Geometry: final body of the model. Coordinates: model frame, mm. A direction names the side the tool comes from. Give positions to 0.01 mm unless a question says otherwise; leave off trailing zeros. Loops run counter-clockwise (first coordinate to the right, second up) from the corner with the lowest first, then second, coordinate; pieces in that order, holes last. Notation, with made-up numbers: M 75.5,9 L 132.5,9 A4 ccw 132.5,15 Z; hole C -13.75,43 d10. An arc over 180 degrees is marked long. Put each result on its own line as item: value.
Autodesk Fusion 360 part; units mm, degrees
sketch "Sketch1" plane through (0, 0, 0) normal (0, 0, 1) x (1, 0, 0)
  circle A0 centre (0, 0) radius 1.75
  dimension "d1" = 3.5
extrude "Extrude1" add sketch "Sketch1" along normal blind 0.3
sketch "Sketch2" plane through (0, 0, 0.3) normal (0, 0, 1) x (-1, 0, 0)
  circle A0 centre (0, 0) radius 1.75
  circle A1 centre (0, 0) radius 1.25
  dimension "d4" = 2.5
extrude "Extrude2" add sketch "Sketch2" along normal blind 2 contours A1
chamfer "Chamfer1" distance 0.4 angle 45 1 edges at (1.1654, 0.452, 2.3)

Autodesk Fusion 360 part; units mm, degrees
sketch "Sketch1" plane through (0, 0, 0) normal (0, 0, 1) x (1, 0, 0)
  line L0 (-26.5, 26.5) -> (26.5, 26.5)
  line L1 (26.5, 26.5) -> (26.5, -26.5)
  line L2 (26.5, -26.5) -> (-26.5, -26.5)
  line L3 (-26.5, -26.5) -> (-26.5, 26.5)
  line L4 (-26.5, 26.5) -> (26.5, -26.5) construction
  line L5 (26.5, 26.5) -> (-26.5, -26.5) construction
  line L6 (-15.8934, 26.5) -> (-26.5, 15.8934)
  line L7 (15.8934, 26.5) -> (26.5, 15.8934)
  line L8 (26.5, -15.8934) -> (15.8934, -26.5)
  line L9 (-26.5, -15.8934) -> (-15.8934, -26.5)
  dimension "d34" = 53
  dimension "d35" = 53
  dimension "d36" = 15
  dimension "d37" = 15
  dimension "d38" = 15
  dimension "d39" = 15
extrude "Extrude1" add sketch "Sketch1" along normal blind 1 contours L0 L1 L2 L3 L6 L7 L8 L9
sketch "Sketch3" plane through (0, 0, 1) normal (0, 0, 1) x (-1, 0, 0)
  line L0 (15.8934, -26.5) -> (26.5, -15.8934)
  line L1 (26.5, -15.8934) -> (26.5, 15.8934)
  line L2 (26.5, 15.8934) -> (15.8934, 26.5)
  line L3 (15.8934, 26.5) -> (-15.8934, 26.5)
  line L4 (-15.8934, 26.5) -> (-26.5, 15.8934)
  line L5 (-26.5, 15.8934) -> (-26.5, -15.8934)
  line L6 (-26.5, -15.8934) -> (-15.8934, -26.5)
  line L7 (-15.8934, -26.5) -> (15.8934, -26.5)
  line L8 (25.5, -25.5) -> (-25.5, -25.5)
  line L9 (-25.5, -25.5) -> (-25.5, 25.5)
  line L10 (-25.5, 25.5) -> (25.5, 25.5)
  line L11 (25.5, 25.5) -> (25.5, -25.5)
  line L12 (25.5, -25.5) -> (-25.5, 25.5) construction
  line L13 (-25.5, -25.5) -> (25.5, 25.5) construction
  line L14 (15.4792, -25.5) -> (25.5, -15.4792)
  line L15 (-15.4792, -25.5) -> (-25.5, -15.4792)
  line L16 (-25.5, 15.4792) -> (-15.4792, 25.5)
  line L17 (15.4792, 25.5) -> (25.5, 15.4792)
  dimension "d42" = 1
  dimension "d43" = 1
  dimension "d44" = 1
  dimension "d45" = 1
  dimension "d46" = 1
extrude "Extrude3" add sketch "Sketch3" along normal blind 13 contours L0 L6 L7 L8 | L0 L8 L11 L14 | L0 L1 L2 L11 | L6 L8 L9 L15 | L4 L5 L6 L9 | L2 L10 L11 L17 | L2 L3 L4 L10 | L4 L9 L10 L16
sketch "Sketch5" plane through (21.1967, -21.1967, 0) normal (0.7071, -0.7071, 0) x (0.7071, 0.7071, 0)
  line L0 (-7.5, 0) -> (7.5, 0)
  line L1 (7.5, 0) -> (7.5, 14)
  line L2 (7.5, 14) -> (-7.5, 14)
  line L3 (-7.5, 14) -> (-7.5, 0)
  line L4 (-2.746, 8.1279) -> (3.1066, 8.15)
  arc A0 (3.1066, 8.15) -> (3.0934, 11.65) centre (3.1, 9.9) ccw
  line L5 (3.0934, 11.65) -> (-2.7592, 11.6279)
  arc A1 (-2.7592, 11.6279) -> (-2.746, 8.1279) centre (-2.7526, 9.8779) ccw
  line L6 (-2.7526, 9.8779) -> (3.1, 9.9) construction
  dimension "d93" = 4.1221
  dimension "d94" = 4.7474
  dimension "d95" = 1.75
  dimension "d96" = 5.8526
extrude "Extrude5" cut sketch "Sketch5" against normal blind 2 contours L4 A0 L5 A1
sketch "Sketch7" plane through (0, 26.5, 0) normal (0, 1, 0) x (-1, 0, 0)
  line L0 (-15.8934, 0) -> (15.8934, 0)
  line L1 (15.8934, 0) -> (15.8934, 14)
  line L2 (15.8934, 14) -> (-15.8934, 14)
  line L3 (-15.8934, 14) -> (-15.8934, 0)
  line L4 (-2.0165, 11.171) -> (2.0293, 11.171)
  line L5 (2.0293, 11.171) -> (2.0293, 8.1421)
  line L6 (2.0293, 8.1421) -> (-2.0165, 8.1421)
  line L7 (-2.0165, 8.1421) -> (-2.0165, 11.171)
  dimension "d82" = 2.829
  dimension "d83" = 4.0458
  dimension "d84" = 3.0289
  dimension "d85" = 13.8769
extrude "Extrude7" cut sketch "Sketch7" along normal through all contours L4 L5 L6 L7
sketch "Sketch8" plane through (-26.5, 0, 0) normal (-1, 0, 0) x (0, -1, 0)
  line L0 (-15.8934, 0) -> (15.8934, 0)
  line L1 (15.8934, 0) -> (15.8934, 14)
  line L2 (15.8934, 14) -> (-15.8934, 14)
  line L3 (-15.8934, 14) -> (-15.8934, 0)
  line L4 (-2.0152, 11.1757) -> (2.0191, 11.1757)
  line L5 (2.0191, 11.1757) -> (2.0191, 8.2313)
  line L6 (2.0191, 8.2313) -> (-2.0152, 8.2313)
  line L7 (-2.0152, 8.2313) -> (-2.0152, 11.1757)
  dimension "d87" = 2.8243
  dimension "d88" = 2.9444
  dimension "d89" = 4.0342
  dimension "d90" = 13.8782
extrude "Extrude8" cut sketch "Sketch8" along normal through all contours L4 L5 L6 L7
sketch "Sketch9" plane through (0, 0, 1) normal (0, 0, 1) x (-1, 0, 0)
  line L0 (25.5, -15.4792) -> (25.5, 15.4792)
  line L1 (25.5, 15.4792) -> (15.4792, 25.5)
  line L2 (15.4792, 25.5) -> (-15.4792, 25.5)
  line L3 (-15.4792, 25.5) -> (-25.5, 15.4792)
  line L4 (-25.5, 15.4792) -> (-25.5, -15.4792)
  line L5 (-25.5, -15.4792) -> (-15.4792, -25.5)
  line L6 (-15.4792, -25.5) -> (15.4792, -25.5)
  line L7 (15.4792, -25.5) -> (25.5, -15.4792)
  circle A0 centre (-9.009, 22.5618) radius 1.1
  circle A1 centre (9.0089, 22.5618) radius 1.1
  circle A2 centre (-9.009, -22.5547) radius 1.1
  circle A3 centre (9.0089, -22.5547) radius 1.1
  dimension "d62" = 2.2
  dimension "d63" = 2.2
  dimension "d64" = 2.2
  dimension "d65" = 2.2
extrude "Extrude9" cut sketch "Sketch9" against normal blind 10 contours A0 | A1 | A2 | A3
chamfer "Chamfer1" distance 1 angle 45 4 edges at (-7.9834, 22.9525, 0) (10.0345, 22.9525, 0) (10.0345, -22.164, 0) (-7.9834, -22.164, 0)
sketch "Sketch11" plane through (-21.1967, -21.1967, 0) normal (-0.7071, -0.7071, 0) x (0.7071, -0.7071, 0)
  line L0 (-7.5, 0) -> (7.5, 0)
  line L1 (7.5, 0) -> (7.5, 14)
  line L2 (7.5, 14) -> (-7.5, 14)
  line L3 (-7.5, 14) -> (-7.5, 0)
  circle A0 centre (0.0835, 9.893) radius 1.5
  dimension "d73" = 3
  dimension "d91" = 4.107
  dimension "d92" = 7.5835
extrude "Extrude11" cut sketch "Sketch11" against normal blind 5 contours A0
sketch "Sketch12" plane through (-20.4896, -20.4896, 0) normal (0.7071, 0.7071, 0) x (-0.7071, 0.7071, 0)
  circle A0 centre (-0.0835, 9.893) radius 1.5
  line L0 (-7.0858, 1) -> (7.0858, 1)
  line L1 (7.0858, 1) -> (7.0858, 14)
  line L2 (7.0858, 14) -> (-7.0858, 14)
  line L3 (-7.0858, 14) -> (-7.0858, 1)
  circle A1 centre (-0.0835, 9.893) radius 1.5
  circle A2 centre (-0.0835, 9.893) radius 2
  dimension "d77" = 4
extrude "Extrude12" cut sketch "Sketch12" against normal blind 0.5 contours A2
sketch "Sketch13" plane through (0, 0, 0) normal (0, 0, -1) x (1, 0, 0)
  circle A0 centre (9.009, 22.5618) radius 2.1
  circle A1 centre (-9.0089, -22.5547) radius 2.1
  line L0 (-26.5, -15.8934) -> (-15.8934, -26.5)
  line L1 (-15.8934, -26.5) -> (15.8934, -26.5)
  line L2 (15.8934, -26.5) -> (26.5, -15.8934)
  line L3 (26.5, -15.8934) -> (26.5, 15.8934)
  line L4 (26.5, 15.8934) -> (15.8934, 26.5)
  line L5 (15.8934, 26.5) -> (-15.8934, 26.5)
  line L6 (-15.8934, 26.5) -> (-26.5, 15.8934)
  line L7 (-26.5, 15.8934) -> (-26.5, -15.8934)
  circle A2 centre (9.009, -22.5547) radius 2.1
  circle A3 centre (-9.0089, 22.5618) radius 2.1
sketch "Sketch14" plane through (0, 0, 1) normal (0, 0, 1) x (-1, 0, 0)
  line L0 (25.5, -15.4792) -> (25.5, 15.4792)
  line L1 (25.5, 15.4792) -> (15.4792, 25.5)
  line L2 (15.4792, 25.5) -> (-15.4792, 25.5)
  line L3 (-15.4792, 25.5) -> (-25.5, 15.4792)
  line L4 (-25.5, 15.4792) -> (-25.5, -15.4792)
  line L5 (-25.5, -15.4792) -> (-15.4792, -25.5)
  line L6 (-15.4792, -25.5) -> (15.4792, -25.5)
  line L7 (15.4792, -25.5) -> (25.5, -15.4792)
  circle A0 centre (9.0089, -22.5547) radius 1.1
  circle A1 centre (9.0089, -22.5547) radius 2.75
  circle A2 centre (-9.009, -22.5547) radius 1.1
  circle A3 centre (-9.009, -22.5547) radius 2.75
  circle A4 centre (9.0089, 22.5618) radius 1.1
  circle A5 centre (9.0089, 22.5618) radius 2.75
  circle A6 centre (-9.009, 22.5618) radius 1.1
  circle A7 centre (-9.009, 22.5618) radius 2.75
  circle A8 centre (9.0089, 22.5618) radius 1.1
  circle A9 centre (9.0089, -22.5547) radius 1.1
  circle A10 centre (-9.009, 22.5618) radius 1.1
  circle A11 centre (-9.009, -22.5547) radius 1.1
  dimension "d97" = 5.5
  dimension "d98" = 5.5
  dimension "d99" = 5.5
  dimension "d100" = 5.5
extrude "Extrude13" add sketch "Sketch14" along normal blind 5.5 contours A1 | A3 | A5 | A7
Item 1: Section C-C on y = -3. Output: boundary loops of the cut face in (x, z), then the cut area to 3 significant figures.
Output values:
outline: M -26.5,0 L 26.5,0 L 26.5,14 L 25.5,14 L 25.5,1 L -25.5,1 L -25.5,14 L -26.5,14 Z
area: 79.0 mm²
Item 2: Pin query (flat end, axial travel): pin 1 Ø2 at (x, y) = (8.5, 15) entering from -Z; pin 2 Ø3 at (x, y) = (8.5, -22.5) entering from +Z; pin 3 Ø8 at (x, z) = (-21, 8) entering from +Y; pin 4 Ø2.5 at (x, y) = (-9.01, 22.55) entering from -Z (3 decimals). Return the tip coordinate at first contact, or that it passes through.
Output values:
pin 1: z = 0
pin 2: z = 6.5
pin 3: y = 25.39
pin 4: z = 0.845
Item 3: Section B-B on x = 0. Output: boundary loops of the cut face in (y, z).
Output values:
outline: M -26.5,0 L 26.5,0 L 26.5,14 L 25.5,14 L 25.5,1 L 1.25,1 L 1.25,1.9 L 0.85,2.3 L -0.85,2.3 L -1.25,1.9 L -1.25,1 L -25.5,1 L -25.5,14 L -26.5,14 Z
Item 4: Section A-A on z = 4.75. Count the separate pieces of the cut face and the enclosed holes in it, then the cut area to 3 significant figures.
Output values:
separate pieces: 5
enclosed holes: 5
area: 264 mm²
Item 5: Set-up query: faces 1 (the flat face through (22, -20, 14)), 2 (the cylindrical face through (-20.421, -20.907, 11.876)), 3 (the flat face through (-22, 22, 0.3)), 4 (the flat face through (23, 24, 0.3)), 5 (the cylindrical face through (-8.41, 19.87, 3.71)). Return all of +Z, -Z, +X, -X, +Y, -Y with unobstructed straight access to the full face (end or side cutting, diameter ignored); none if empty.
Output values:
face 1: +Z, +X, -X, +Y, -Y
face 2: none
face 3: +Z, -X, +Y
face 4: +Z, +X, +Y
face 5: +Z
Item 6: Mould query, pull axis Y, two halves, no side actions, for faces 6 (the flat face through (-24, -23, 0.3)), 7 (the flat face through (5, 0, 1)), 8 (the flat face through (21.122, 21.271, 7.054)). Classes: pulls with the +Y half, pulls with the -Y half, needs draft (parallel to the pull), parting line crosses it, or undercut.
Output values:
face 6: needs draft
face 7: undercut
face 8: pulls with the +Y half
Item 7: Line query: probe 1 along X at (y, z) = (5.5, 6.25); probe 2 along X at (y, z) = (22, 6.25). Output: solid intervals per line, ascending. Write a range as [from, to].
Output values:
probe 1: [-26.5, -25.5], [25.5, 26.5]
probe 2: [-20.39, -18.98], [-11.7, -9.96], [-8.06, -6.32], [6.32, 8.06], [9.96, 11.7], [18.98, 20.39]
